```python
from build123d import *

# Parameters (mm, degrees)
F1_DEPTH = 6.35


with BuildPart() as f1:
    # F0 (on Front) → F1 (new body)
    with BuildSketch(Plane.XZ):
        Polygon((57.603374, 3.126765), (57.052041, 0), (63.5, 0), (64.051333, 3.126765), align=None)
        Polygon((67.910664, 25.014117), (64.602666, 6.253529), (64.051333, 3.126765), (63.5, 0), (88.9, 0), (90.002666, 6.253529), (83.554707, 6.253529), (70.854707, 6.253529), (73.060039, 18.760588), (85.760039, 18.760588), (92.207998, 18.760588), (93.310664, 25.014117), align=None)
        Polygon((4.410664, 25.014117), (0, 0), (6.35, 0), (8.555332, 12.507058), (14.905332, 12.507058), (15.46517, 15.682058), (12.29017, 15.682058), (13.426252, 21.935588), (16.567836, 21.935588), (17.110664, 25.014117), align=None)
        Polygon((42.510664, 25.014117), (36.160664, 25.014117), (32.309838, 3.175), (31.75, 0), (38.1, 0), (39.202666, 6.253529), align=None)
        Polygon((29.810664, 25.014117), (17.110664, 25.014117), (16.567836, 21.935588), (19.742836, 21.935588), (18.64017, 15.682058), (15.46517, 15.682058), (14.905332, 12.507058), (21.255332, 12.507058), (19.05, 0), (25.4, 0), (25.959838, 3.175), align=None)
        Polygon((32.309838, 3.175), (25.959838, 3.175), (25.4, 0), (31.75, 0), align=None)
        Polygon((58.154707, 6.253529), (39.202666, 6.253529), (38.1, 0), (57.052041, 0), (57.603374, 3.126765), align=None)
    extrude(amount=F1_DEPTH)


solid = f1.part
```
Geometry: final body of the model. Coordinates: model frame, mm. A direction names the side the tool comes from. Round coordinates to 2 decimals unless told otherwise and drop trailing zeros. Write each loop counter-clockwise with the first axis right and the second up, starting at its lowest first coordinate (ties: lowest second). Pieces come first, ordered by that corner, then holes. Notation, with made-up numbers: (56.5, 81.25) -> (69.5, 81.25) arc R18 ccw to (69.5, 92.25) -> close; hole circle Ø6 at (77, 15). An arc over 180 degrees is marked (long way). Use CSV: the item, a comma, the result in double quotes. Start each with the question number.
Q1. Reachability of faces 5 (the face through (20.168, -3.131, 6.341)), 6 (the face through (81, -3, 6.254)), 7 (the face through (39, -3, 25.014)) from +Z, -Z, +X, -X, +Y, -Y: full face, straight path, thin tool, end or side. Return the list, or none.
Q2. Section C-C (z = 13.75). Return loops of the section in (x, y), plus the area to 3 significant figures.
Q3. Section A-A (x = 80). Return loops of the section in (y, z), plus the area to 3 significant figures.
Q4. First-contact query: pin 1 Ø3 at (x, y) = (46, -4.5) entering from +Z; pin 2 Ø10 at (x, z) = (10, 3) entering from -Y; pin 3 Ø1.9 at (x, y) = (15.5, -3) entering from -Z; pin 4 Ø3 at (y, z) = (-1.5, 9) entering from +X. Flat tips, straight axial feed; report the tip coordinate or a pass-through.
Q5. Section D-D (z = 9). Return loops of the section in (x, y).
Q6. Section B-B (y = -2.25). Return loops of the section in (x, z) (3 decimals).
Q7. Pull-direction query (Z, two-part tool) for faces 1 (the face through (16, -3, 15.682)), 2 (the face through (36, 0, 13)), 3 (the face through (34.262, -3.131, 14.247)), 4 (the face through (92.75, -3.13, 21.84)); classes: pulls with the +Z half, pulls with the -Z half, needs draft (parallel to the pull), parting line crosses it, or undercut.
Q8. Line query: L1, parallel to Z at x = 80, y = -4.25; L2, parallel to X at y = -1.5, z = 11.5; L3, parallel to X at y = -4, z = 22.75. Output: solid intervals per line, ascending.
Result sheet:
1,face 5,"+Y, -Y"
1,face 6,"+X, +Y, -Y"
1,face 7,"+Z, +X, -X, +Y, -Y"
2,outline,"(2.42, -6.35) -> (27.82, -6.35) -> (27.82, 0) -> (2.42, 0) -> close; (34.17, -6.35) -> (40.52, -6.35) -> (40.52, 0) -> (34.17, 0) -> close; (65.92, -6.35) -> (72.18, -6.35) -> (72.18, 0) -> (65.92, 0) -> close"
2,area,"241 mm²"
3,outline,"(-6.35, 0) -> (0, 0) -> (0, 6.25) -> (-6.35, 6.25) -> close; (-6.35, 18.76) -> (0, 18.76) -> (0, 25.01) -> (-6.35, 25.01) -> close"
3,area,"79.4 mm²"
4,pin 1,"z = 6.25"
4,pin 2,"y = -6.35"
4,pin 3,"z = 12.51"
4,pin 4,"x = 71.6"
5,outline,"(1.59, -6.35) -> (7.94, -6.35) -> (7.94, 0) -> (1.59, 0) -> close; (20.64, -6.35) -> (26.99, -6.35) -> (26.99, 0) -> (20.64, 0) -> close; (33.34, -6.35) -> (39.69, -6.35) -> (39.69, 0) -> (33.34, 0) -> close; (65.09, -6.35) -> (71.34, -6.35) -> (71.34, 0) -> (65.09, 0) -> close"
6,outline,"(0, 0) -> (6.35, 0) -> (8.555, 12.507) -> (21.255, 12.507) -> (19.05, 0) -> (88.9, 0) -> (90.003, 6.254) -> (70.855, 6.254) -> (73.06, 18.761) -> (92.208, 18.761) -> (93.311, 25.014) -> (67.911, 25.014) -> (64.051, 3.127) -> (57.603, 3.127) -> (58.155, 6.254) -> (39.203, 6.254) -> (42.511, 25.014) -> (36.161, 25.014) -> (32.31, 3.175) -> (25.96, 3.175) -> (29.811, 25.014) -> (4.411, 25.014) -> close; hole (12.29, 15.682) -> (18.64, 15.682) -> (19.743, 21.936) -> (13.426, 21.936) -> close"
7,face 1,"undercut"
7,face 2,"needs draft"
7,face 3,"pulls with the +Z half"
7,face 4,"pulls with the -Z half"
8,L1,"0 to 6.25, 18.76 to 25.01"
8,L2,"2.03 to 8.38, 21.08 to 27.43, 33.78 to 40.13, 65.53 to 71.78"
8,L3,"4.01 to 29.41, 35.76 to 42.11, 67.51 to 92.91"
